Check sheet for the modelled part. Datum: model origin and axes. Units: mm. A direction names the side the tool comes from. Coordinates: 2 decimals unless noted, no trailing zeros. Write each loop counter-clockwise with the first axis right and the second up, starting at its lowest first coordinate (ties: lowest second). Pieces come first, ordered by that corner, then holes. Notation, with made-up numbers: (79, 22.25) - (91, 22.25) arc R26 cw to (91, 37.25) - close; hole circle Ø6 at (20, -6.75). An arc over 180 degrees is marked (long way). Write each question's results on one line, items separated by ' | '.
from build123d import *

# Parameters (mm, degrees)
SCHIZZO1_W                        = 41
SCHIZZO1_H                        = 20
ESTRUSIONE_ESTRUSIONE1_DEPTH      = 43
SCHIZZO2_R                        = 3
ESTRUSIONE_ESTRUSIONE4_DEPTH      = 4
ESTRUSIONE_ESTRUSIONE5_DEPTH      = 10
ESTRUSIONE_ESTRUSIONE5_DEPTH_BACK = 10
SCHIZZO4_W                        = 54
SCHIZZO4_H                        = 2.5
FORO_PER_VITE_M1_6_1_D            = 4.5


with BuildPart() as part:
    # Schizzo1 → Estrusione-Estrusione1 (new body)
    with BuildSketch(Plane(origin=(0, 0, 0), x_dir=(1, 0, 0), z_dir=(0, 1, 0))):
        with Locations((10.5, 0)):
            Rectangle(SCHIZZO1_W, SCHIZZO1_H)
    extrude(amount=ESTRUSIONE_ESTRUSIONE1_DEPTH)

    # Schizzo2 → Estrusione-Estrusione4 (add)
    with BuildSketch(Plane(origin=(0, 43, 0), x_dir=(1, 0, 0), z_dir=(0, 1, 0))):
        with Locations(Location((0, 0, 0), (0, 0, 270))):
            Circle(SCHIZZO2_R)
    extrude(amount=ESTRUSIONE_ESTRUSIONE4_DEPTH)

    # Schizzo4 → Estrusione-Estrusione5 (add, two sides: drawn at the far end of the back side and taken through both)
    with BuildSketch(Plane.XY.offset(-ESTRUSIONE_ESTRUSIONE5_DEPTH_BACK)):
        with Locations((10.5, 25.75)):
            Rectangle(SCHIZZO4_W, SCHIZZO4_H)
    extrude(amount=ESTRUSIONE_ESTRUSIONE5_DEPTH + ESTRUSIONE_ESTRUSIONE5_DEPTH_BACK)

    # Foro per Vite M1.6-1 (through all)
    with Locations(Plane(origin=(0, 27, 0), x_dir=(1, 0, 0), z_dir=(0, 1, 0))):
        with Locations((-13.250292536, 5), (-13.250292536, -5), (34.250292536, 5), (34.250292536, -5)):
            Hole(FORO_PER_VITE_M1_6_1_D / 2)


solid = part.part
1. Material ranges on L1, parallel to Y at x = 15, z = 7; L2, parallel to Y at x = -13, z = -2.5; L3, parallel to X at y = 42, z = -5.75, recorded low to high. Write a range as [from, to].
Values follow:
L1: y = [0, 43] | L2: y = [24.5, 27] | L3: x = [-10, 31]
2. Sectioned sample at A-A (z = 5). Record the cut outline in (x, y), then the cut area to 3 significant figures.
Values follow:
outline: (-16.5, 24.5) - (-15.5, 24.5) - (-15.5, 27) - (-16.5, 27) - close; (-11, 24.5) - (-10, 24.5) - (-10, 0) - (31, 0) - (31, 24.5) - (32, 24.5) - (32, 27) - (31, 27) - (31, 43) - (-10, 43) - (-10, 27) - (-11, 27) - close; (36.5, 24.5) - (37.5, 24.5) - (37.5, 27) - (36.5, 27) - close | area: 1,770 mm^2
3. Sectioned sample at D-D (y = 31.5). Record the cut outline in (x, z).
Values follow:
outline: (-10, -10) - (31, -10) - (31, 10) - (-10, 10) - close
4. Go/stop test with flat-tipped pins: pin 1 (3.5 mm diameter, centred on x = -13.25, z = 5, fed in from +Y); pin 2 (3 mm diameter, centred on x = 34.5, z = 1, fed in from +Y); pin 3 (1 mm diameter, centred on x = -2, z = -3, fed in from +Y); pin 4 (8 mm diameter, centred on y = 20, z = -6, fed in from +X). Record where each tip stops, or that it passes through.
Values follow:
pin 1: passes through | pin 2: stops at y = 27 | pin 3: stops at y = 43 | pin 4: stops at x = 31
5. Sectioned sample at C-C (x = 0). Record the cut outline in (y, z).
Values follow:
outline: (0, -10) - (43, -10) - (43, -3) - (47, -3) - (47, 3) - (43, 3) - (43, 10) - (0, 10) - close
6. Access from +Z, -Z, +X, -X, +Y, -Y to the whole of each face (thin tool, end or side, straight path). Record for faces 4 (the flat face through (34, 24.5, 0)), 5 (the flat face through (-10, 12, 0)), 6 (the flat face through (-13, 27, 0)).
Values follow:
face 4: +Z, -Z, +X, -Y | face 5: +Z, -Z, -X, -Y | face 6: +Z, -Z, -X, +Y
7. Draft check along Z on faces 1 (the flat face through (34, 27, 0)), 2 (the cylindrical face through (32.17, 25.73, 5.86)), 3 (the cylindrical face through (0.9, 44.97, 2.86)). Enter one of: pulls with the +Z half, pulls with the -Z half, needs draft (parallel to the pull), parting line crosses it, or undercut.
Values follow:
face 1: needs draft | face 2: undercut | face 3: parting line crosses it
8. Sectioned sample at B-B (z = 0). Record the cut outline in (x, y), then the cut area to 3 significant figures.
Values follow:
outline: (-16.5, 24.5) - (-10, 24.5) - (-10, 0) - (31, 0) - (31, 24.5) - (37.5, 24.5) - (37.5, 27) - (31, 27) - (31, 43) - (3, 43) - (3, 47) - (-3, 47) - (-3, 43) - (-10, 43) - (-10, 27) - (-16.5, 27) - close | area: 1,820 mm^2
